Can you work these out from the drawing? Everything is in mm from the part's minimum corner. A direction names the side the tool comes from. Coordinates: 2 decimals unless noted, no trailing zeros. Loops run counter-clockwise (first coordinate to the right, second up) from the corner with the lowest first, then second, coordinate; pieces in that order, holes last. Notation, with made-up numbers: (-38.5, 39.5) -> (19.5, 39.5) arc R8 cw to (19.5, 51.5) -> close; hole circle Ø10 at (2.5, -6.5). An arc over 180 degrees is marked (long way). One line per question, with ' | ' between items.
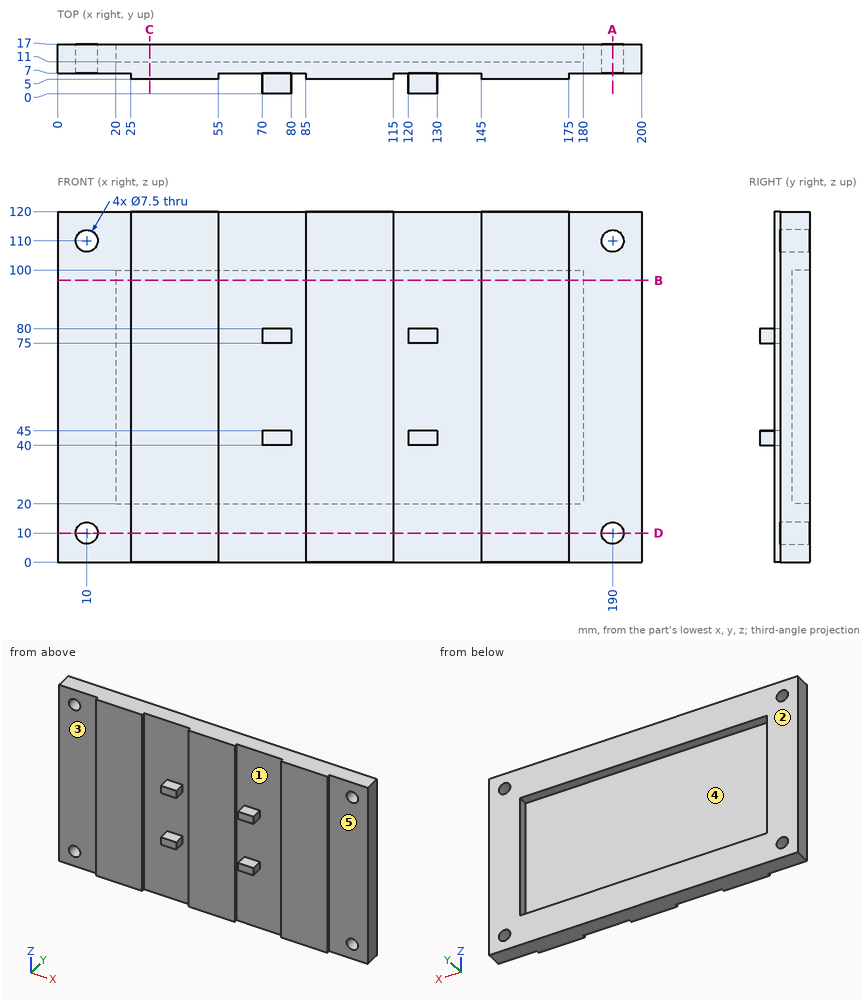
Q1. For pin 1 (10 mm diameter, centred on x = 77, z = 47.5, fed in from -Y); pin 2 (1 mm diameter, centred on x = 59, z = 70.5, fed in from +Y); pin 3 (15 mm diameter, centred on x = 34, z = 54.5, fed in from -Y); pin 4 (0.6 mm diameter, centred on y = 5.5, z = 32, fed in from +X), each with a flat end and sliding along its axis, tell me the tip position at first contact or that it passes through.
Values follow:
pin 1: stops at y = 0 | pin 2: stops at y = 11 | pin 3: stops at y = 5 | pin 4: stops at x = 175
Q2. We'd pull the mould along X, two halves only. Please class the marked faces 1 and 2: released by +X, released by -X, zero draft, split by the parting line, or undercut.
Values follow:
face 1: undercut | face 2: zero draft
Q3. Imagine slicing it at C-C on x = 31.5. Write out the boundary of the cut face in (y, z), plus the area to 3 significant figures.
Values follow:
outline: (5, 0) -> (17, 0) -> (17, 20) -> (11, 20) -> (11, 100) -> (17, 100) -> (17, 120) -> (5, 120) -> close | area: 960 mm2
Q4. Imagine slicing it at A-A on x = 190. Write out the boundary of the cut face in (y, z), plus the area to 3 significant figures.
Values follow:
outline: (7, 0) -> (17, 0) -> (17, 6.25) -> (7, 6.25) -> close; (7, 13.75) -> (17, 13.75) -> (17, 106.25) -> (7, 106.25) -> close; (7, 113.75) -> (17, 113.75) -> (17, 120) -> (7, 120) -> close | area: 1,050 mm2
Q5. Imagine slicing it at B-B on z = 96.5. Write out the boundary of the cut face in (x, y).
Values follow:
outline: (0, 7) -> (25, 7) -> (25, 5) -> (55, 5) -> (55, 7) -> (85, 7) -> (85, 5) -> (115, 5) -> (115, 7) -> (145, 7) -> (145, 5) -> (175, 5) -> (175, 7) -> (200, 7) -> (200, 17) -> (180, 17) -> (180, 11) -> (20, 11) -> (20, 17) -> (0, 17) -> close
Q6. Imagine slicing it at D-D on z = 10. Write out the boundary of the cut face in (x, y).
Values follow:
outline: (0, 7) -> (6.25, 7) -> (6.25, 17) -> (0, 17) -> close; (13.75, 7) -> (25, 7) -> (25, 5) -> (55, 5) -> (55, 7) -> (85, 7) -> (85, 5) -> (115, 5) -> (115, 7) -> (145, 7) -> (145, 5) -> (175, 5) -> (175, 7) -> (186.25, 7) -> (186.25, 17) -> (13.75, 17) -> close; (193.75, 7) -> (200, 7) -> (200, 17) -> (193.75, 17) -> close
Q7. For the marked faces 3, 4 and 5, which set-ups out of +Z, -Z, +X, -X, +Y, -Y let a thin tool reach every point of the face, with its end or its side?
Values follow:
face 3: +Z, -Z, -X, -Y | face 4: +Y | face 5: +Z, -Z, +X, -Y
Q8. Please list where these lines run through material, in increasing order: L1, parallel to X at y = 14.5, z = 110; L2, parallel to Z at x = 190, y = 14; L3, parallel to X at y = 6.5, z = 65. Write a range as [from, to].
Values follow:
L1: x = [0, 6.25], [13.75, 186.25], [193.75, 200] | L2: z = [0, 6.25], [13.75, 106.25], [113.75, 120] | L3: x = [25, 55], [85, 115], [145, 175]
